The figure shows three views and two pictorial views of one solid part (mm, origin at its lowest corner). Answer the questions. Give positions to 0.01 mm unless a question says otherwise; leave off trailing zeros. Loops run counter-clockwise (first coordinate to the right, second up) from the corner with the lowest first, then second, coordinate; pieces in that order, holes last. Notation, with made-up numbers: (52, 38) - (102, 38) arc R11 cw to (102, 50) - close; hole circle Ø7 at (-0.75, 11.5). An arc over 180 degrees is marked (long way). Use CSV: the item, a comma, the result in double quotes.
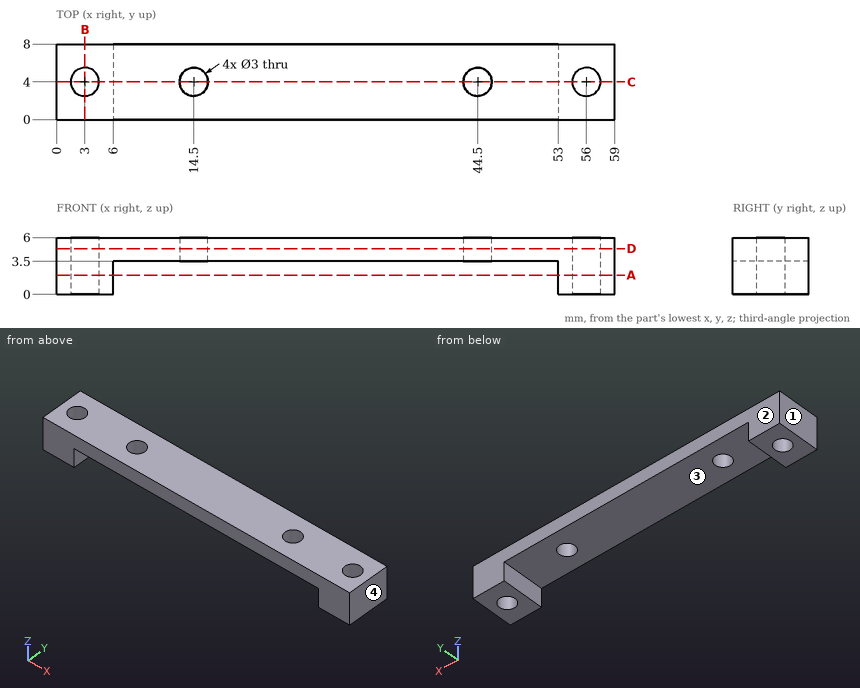
Item 1: A cutting plane is placed at C-C on y = 4. Determine the outline of the cut face in (x, z), and give its area (4 significant figures).
Determined:
outline,"(0, 0) - (1.5, 0) - (1.5, 6) - (0, 6) - close; (4.5, 0) - (6, 0) - (6, 3.5) - (13, 3.5) - (13, 6) - (4.5, 6) - close; (16, 3.5) - (43, 3.5) - (43, 6) - (16, 6) - close; (46, 3.5) - (53, 3.5) - (53, 0) - (54.5, 0) - (54.5, 6) - (46, 6) - close; (57.5, 0) - (59, 0) - (59, 6) - (57.5, 6) - close"
area,"138.5 mm²"
Item 2: A cutting plane is placed at A-A on z = 2.05. Determine the outline of the cut face in (x, y), and give its area (3 significant figures).
Determined:
outline,"(0, 0) - (6, 0) - (6, 8) - (0, 8) - close; (53, 0) - (59, 0) - (59, 8) - (53, 8) - close; hole circle Ø3 at (3, 4); hole circle Ø3 at (56, 4)"
area,"81.9 mm²"
Item 3: Find the intervals of material crossed by line 1 (X direction, y = 5.75, z = 1.5); line 2 (Y direction, x = 56, z = 1.55); line 3 (X direction, y = 3.5, z = 2.7), in increasing order.
Determined:
line 1,"x = 0 to 6, 53 to 59"
line 2,"y = 0 to 2.5, 5.5 to 8"
line 3,"x = 0 to 1.59, 4.41 to 6, 53 to 54.59, 57.41 to 59"
Item 4: Given P1, Ø2, axis at x = 46.5, y = 2.5, coming from the -Z side, flat-ended and moving along its own axis, determine where the tip first touches the part or whether it passes through.
Determined:
P1,"stops at z = 3.5"
Item 5: A cutting plane is placed at D-D on z = 4.85. Determine the outline of the cut face in (x, y).
Determined:
outline,"(0, 0) - (59, 0) - (59, 8) - (0, 8) - close; hole circle Ø3 at (3, 4); hole circle Ø3 at (14.5, 4); hole circle Ø3 at (44.5, 4); hole circle Ø3 at (56, 4)"
Item 6: A cutting plane is placed at B-B on x = 3. Determine the outline of the cut face in (y, z).
Determined:
outline,"(0, 0) - (2.5, 0) - (2.5, 6) - (0, 6) - close; (5.5, 0) - (8, 0) - (8, 6) - (5.5, 6) - close"
Item 7: The mould has two halves that part along X. Classify the marked faces 1, 2, 3 and 4: pulls with the +X half, pulls with the -X half, needs draft (parallel to the pull), parting line crosses it, or undercut.
Determined:
face 1,"pulls with the -X half"
face 2,"needs draft"
face 3,"undercut"
face 4,"pulls with the +X half"
